```python
from build123d import *

# Parameters (mm, degrees)
F0_R     = 10.25
F0_R_2   = 8.25
F1_DEPTH = 0.5
F2_W     = 20.5
F2_H     = 20.5
F3_DEPTH = 4


with BuildPart() as f1:
    # F0 (on Top) → F1 (new body)
    with BuildSketch(Plane.XY):
        Circle(F0_R)
        Circle(F0_R_2, mode=Mode.SUBTRACT)
    extrude(amount=F1_DEPTH)

    # F2 (on face) → F3 (join)
    with BuildSketch(Plane.XY.offset(0.5)):
        Rectangle(F2_W, F2_H)
    extrude(amount=F3_DEPTH)


solid = f1.part
```
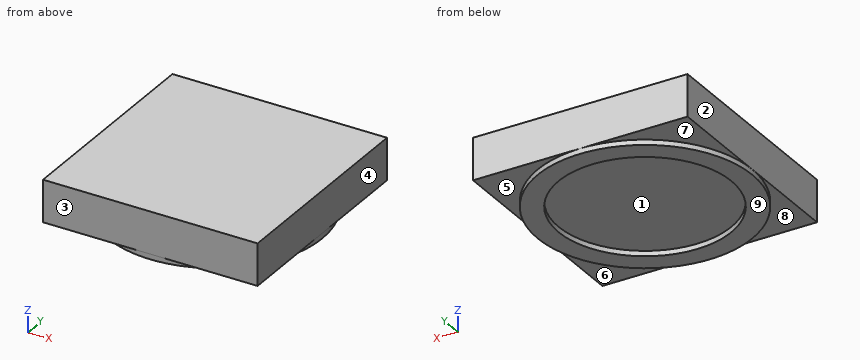
The model under review builds one solid part; all positions refer to its coordinate system, in mm. Face numbers are marked on the shaded views. A direction names the side the tool comes from. Round coordinates to 2 decimals unless told otherwise and drop trailing zeros. Write each loop counter-clockwise with the first axis right and the second up, starting at its lowest first coordinate (ties: lowest second). Pieces come first, ordered by that corner, then holes. Notation, with made-up numbers: (-28, -13) - (18, -13) arc R28 cw to (18, 25) - close; hole circle Ø6 at (18, 23). An arc over 180 degrees is marked (long way). One line per question, with ' | ' between items.
Item 1: Add section B-B, the plane y = 9. Give the boundary of the cut face in (x, z).
Resolved:
outline: (-10.25, 0.5) - (-4.91, 0.5) - (-4.91, 0) - (4.91, 0) - (4.91, 0.5) - (10.25, 0.5) - (10.25, 4.5) - (-10.25, 4.5) - close
Item 2: Add section A-A, the plane x = 2.5. Give the boundary of the cut face in (y, z), then the cut area to 3 significant figures.
Resolved:
outline: (-10.25, 0.5) - (-9.94, 0.5) - (-9.94, 0) - (-7.86, 0) - (-7.86, 0.5) - (7.86, 0.5) - (7.86, 0) - (9.94, 0) - (9.94, 0.5) - (10.25, 0.5) - (10.25, 4.5) - (-10.25, 4.5) - close | area: 84.1 mm2
Item 3: For P1, Ø5, axis at x = 5, y = 2.5, coming from the -Z side, flat-tipped, find the tip position at first contact; note if it passes through.
Resolved:
P1: stops at z = 0.5
Item 4: For the marked faces 5, 6, 7, 8 and 9, list the 3-axis set-ups (+Z, -Z, +X, -X, +Y, -Y) from which the entire face can be reached by the end or side of a thin tool; tool diameter is ignored.
Resolved:
face 5: -Z, +X, +Y | face 6: -Z, +X, -Y | face 7: -Z, -X, +Y | face 8: -Z, -X, -Y | face 9: -Z, +X, -X, +Y, -Y
Item 5: To check wall thickness, follow probe 1 along Y at (x, z) = (0, 0.25); probe 2 along X at (y, z) = (5, 0.2); probe 3 along Z at (x, y) = (-2.5, -6.5). State the ranges of each line that lie inside material, in increasing order.
Resolved:
probe 1: y = -10.25 to -8.25, 8.25 to 10.25 | probe 2: x = -8.95 to -6.56, 6.56 to 8.95 | probe 3: z = 0.5 to 4.5
Item 6: The part is to be moulded in two halves that separate along X. For the marked faces 1, 2, 3 and 4, say which applies: pulls with the +X half, pulls with the -X half, needs draft (parallel to the pull), parting line crosses it, or undercut.
Resolved:
face 1: undercut | face 2: pulls with the -X half | face 3: needs draft | face 4: pulls with the +X half
Item 7: Add section C-C, the plane y = 4.25. Give the boundary of the cut face in (x, z).
Resolved:
outline: (-10.25, 0.5) - (-9.33, 0.5) - (-9.33, 0) - (-7.07, 0) - (-7.07, 0.5) - (7.07, 0.5) - (7.07, 0) - (9.33, 0) - (9.33, 0.5) - (10.25, 0.5) - (10.25, 4.5) - (-10.25, 4.5) - close
